Design review of the part built by this model. Coordinates are the model's own, in mm. A direction names the side the tool comes from. Give positions to 0.01 mm unless a question says otherwise; leave off trailing zeros. Write each loop counter-clockwise with the first axis right and the second up, starting at its lowest first coordinate (ties: lowest second). Pieces come first, ordered by that corner, then holes.
```python
from build123d import *

# Parameters (mm, degrees)
SKETCH1_W           = 72.4
SKETCH1_H           = 66.6
SKETCH1_R           = 1.75
BOSS_EXTRUDE1_DEPTH = 2
SKETCH2_W           = 72.4
SKETCH2_H           = 66.6
SKETCH2_R           = 1
BOSS_EXTRUDE2_DEPTH = 2
SKETCH3_W           = 72.4
SKETCH3_H           = 66.6
BOSS_EXTRUDE3_DEPTH = 1.5


with BuildPart() as part:
    # Sketch1 → Boss-Extrude1 (new body)
    with BuildSketch(Plane(origin=(0, 0, 0), x_dir=(1, 0, 0), z_dir=(0, 1, 0))):
        with Locations((36.2, 33.3)):
            Rectangle(SKETCH1_W, SKETCH1_H)
        with Locations((18.7, 62.843663413)):
            Circle(SKETCH1_R, mode=Mode.SUBTRACT)
        with Locations((13.45, 4.077708133)):
            Circle(SKETCH1_R, mode=Mode.SUBTRACT)
        with Locations((58.95, 4.077708133)):
            Circle(SKETCH1_R, mode=Mode.SUBTRACT)
        with Locations((53.7, 62.843663413)):
            Circle(SKETCH1_R, mode=Mode.SUBTRACT)
    extrude(amount=BOSS_EXTRUDE1_DEPTH)

    # Sketch2 → Boss-Extrude2 (add)
    with BuildSketch(Plane(origin=(0, 2, 0), x_dir=(1, 0, 0), z_dir=(0, 1, 0))):
        with Locations((36.2, 33.3)):
            Rectangle(SKETCH2_W, SKETCH2_H)
        with Locations((3.7, 3.8)):
            Circle(SKETCH2_R, mode=Mode.SUBTRACT)
        with Locations((68.7, 3.8)):
            Circle(SKETCH2_R, mode=Mode.SUBTRACT)
        with Locations((3.7, 62.8)):
            Circle(SKETCH2_R, mode=Mode.SUBTRACT)
        with BuildLine():
            Line((12.059629936, 2), (4.571779789, 2))
            ThreePointArc((4.571779789, 2), (5.185663494, 5.138956303), (2, 4.853565375))
            Line((2, 4.853565375), (2, 61.746434625))
            ThreePointArc((2, 61.746434625), (5.185663494, 61.461043697), (4.571779789, 64.6))
            Line((4.571779789, 64.6), (16.920876117, 64.6))
            ThreePointArc((16.920876117, 64.6), (18.7, 65.343663413), (20.479123883, 64.6))
            Line((20.479123883, 64.6), (51.920876117, 64.6))
            ThreePointArc((51.920876117, 64.6), (53.7, 65.343663413), (55.479123883, 64.6))
            Line((55.479123883, 64.6), (67.828220211, 64.6))
            ThreePointArc((67.828220211, 64.6), (67.214336506, 61.461043697), (70.4, 61.746434625))
            Line((70.4, 61.746434625), (70.4, 4.853565375))
            ThreePointArc((70.4, 4.853565375), (67.214336506, 5.138956303), (67.828220211, 2))
            Line((67.828220211, 2), (60.340370064, 2))
            ThreePointArc((60.340370064, 2), (58.95, 1.577708133), (57.559629936, 2))
            Line((57.559629936, 2), (14.840370064, 2))
            ThreePointArc((14.840370064, 2), (13.45, 1.577708133), (12.059629936, 2))
        make_face(mode=Mode.SUBTRACT)
        with Locations((68.7, 62.8)):
            Circle(SKETCH2_R, mode=Mode.SUBTRACT)
    extrude(amount=BOSS_EXTRUDE2_DEPTH)

    # Sketch3 → Boss-Extrude3 (add)
    with BuildSketch(Plane(origin=(0, 4, 0), x_dir=(1, 0, 0), z_dir=(0, 1, 0))):
        with Locations((36.2, 33.3)):
            Rectangle(SKETCH3_W, SKETCH3_H)
        with BuildLine():
            Line((12.059629936, 2), (2, 2))
            Line((2, 2), (2, 64.6))
            Line((2, 64.6), (16.920876117, 64.6))
            ThreePointArc((16.920876117, 64.6), (18.7, 65.343663413), (20.479123883, 64.6))
            Line((20.479123883, 64.6), (51.920876117, 64.6))
            ThreePointArc((51.920876117, 64.6), (53.7, 65.343663413), (55.479123883, 64.6))
            Line((55.479123883, 64.6), (70.4, 64.6))
            Line((70.4, 64.6), (70.4, 2))
            Line((70.4, 2), (60.340370064, 2))
            ThreePointArc((60.340370064, 2), (58.95, 1.577708133), (57.559629936, 2))
            Line((57.559629936, 2), (14.840370064, 2))
            ThreePointArc((14.840370064, 2), (13.45, 1.577708133), (12.059629936, 2))
        make_face(mode=Mode.SUBTRACT)
    extrude(amount=BOSS_EXTRUDE3_DEPTH)


solid = part.part
```
(1) Consider section A-A, the plane x = 13.45. Give the boundary of the cut face in (y, z), then the cut area to 3 significant figures.
Resolved:
outline: (0, -66.6) - (5.5, -66.6) - (5.5, -64.6) - (2, -64.6) - (2, -5.83) - (0, -5.83) - close; (0, -2.33) - (2, -2.33) - (2, -1.58) - (5.5, -1.58) - (5.5, 0) - (0, 0) - close
area: 139 mm2
(2) Tool access review of faces 1 (the face through (53.47, 0.99, -64.58)), 2 (the face through (2, 4, -33)): name each direction out of +Z, -Z, +X, -X, +Y, -Y from which nothing blocks a thin tool from reaching the whole face with its end or side.
Resolved:
face 1: +Y, -Y
face 2: +Y
(3) Consider section C-C, the plane x = 3.7. Give the boundary of the cut face in (y, z).
Resolved:
outline: (0, -66.6) - (5.5, -66.6) - (5.5, -64.6) - (4, -64.6) - (4, -63.8) - (2, -63.8) - (2, -61.8) - (4, -61.8) - (4, -60.8) - (2, -60.8) - (2, -5.8) - (4, -5.8) - (4, -4.8) - (2, -4.8) - (2, -2.8) - (4, -2.8) - (4, -2) - (5.5, -2) - (5.5, 0) - (0, 0) - close
(4) Consider section D-D, the plane y = 2.8. Give the boundary of the cut face in (x, z), then the cut area to 3 significant figures.
Resolved:
outline: (0, -66.6) - (72.4, -66.6) - (72.4, 0) - (0, 0) - close; hole (2, -61.75) arc R2 cw (long way) to (4.57, -64.6) - (16.92, -64.6) arc R2.5 ccw to (20.48, -64.6) - (51.92, -64.6) arc R2.5 ccw to (55.48, -64.6) - (67.83, -64.6) arc R2 cw (long way) to (70.4, -61.75) - (70.4, -4.85) arc R2 cw (long way) to (67.83, -2) - (60.34, -2) arc R2.5 ccw to (57.56, -2) - (14.84, -2) arc R2.5 ccw to (12.06, -2) - (4.57, -2) arc R2 cw (long way) to (2, -4.85) - close; hole circle Ø2 at (3.7, -62.8); hole circle Ø2 at (3.7, -3.8); hole circle Ø2 at (68.7, -62.8); hole circle Ø2 at (68.7, -3.8)
area: 571 mm2
(5) Clearance check with flat-ended pins moving along their axes: P1, Ø3, axis at x = 13.45, z = -4.08, coming from the +Y side; P2, Ø2, axis at x = 3.5, z = -4, coming from the +Y side; P3, Ø12, axis at x = 56.5, z = -20, coming from the +Y side. State where each tip first meets the part, or that it passes through.
Resolved:
P1: passes through
P2: stops at y = 4
P3: stops at y = 2
(6) Mouldability with a two-part tool opening along X and no side actions: class faces 3 (the face through (70.4, 4, -34)), 4 (the face through (36, 3, 0)), 5 (the face through (72.4, 3, -33)) as pulls with the +X half, pulls with the -X half, needs draft (parallel to the pull), parting line crosses it, or undercut.
Resolved:
face 3: undercut
face 4: needs draft
face 5: pulls with the +X half
(7) Consider section B-B, the plane z = -39. Give the boundary of the cut face in (x, y).
Resolved:
outline: (0, 0) - (72.4, 0) - (72.4, 5.5) - (70.4, 5.5) - (70.4, 2) - (2, 2) - (2, 5.5) - (0, 5.5) - close
(8) To check wall thickness, follow L1, parallel to Z at x = 68.7, y = 2.95; L2, parallel to X at y = 2.5, z = -3.8; L3, parallel to Z at x = 51.5, y = 4.75. State the ranges of each line that lie inside material, in increasing order.
Resolved:
L1: z = -66.6 to -63.8, -61.8 to -60.8, -5.8 to -4.8, -2.8 to 0
L2: x = 0 to 2.7, 4.7 to 5.7, 66.7 to 67.7, 69.7 to 72.4
L3: z = -66.6 to -64.6, -2 to 0
